The drawing under review shows one solid part. Ordinate dimensions are in mm from its lowest x, y, z. A direction names the side the tool comes from. Give positions to 0.01 mm unless a question says otherwise; leave off trailing zeros. Order: outer loops, then holes, each group sorted by start corner. A loop starts at its lowest first (then second) coordinate and runs counter-clockwise, first axis right, second up. Notation, with made-up numbers: (56, 19) -> (65, 19) arc R30 ccw to (65, 41) -> close; hole circle Ø7 at (-35, 32.5). An arc over 180 degrees is marked (long way). One line per item, written item: value. Start each with the question number.
1) Consider section D-D (x = 10). State the section outline as (y, z) points, plus the area to 3 significant figures.
2) Consider section A-A (x = 30). State the section outline as (y, z) points, plus the area to 3 significant figures.
3) Tool access review of the marked faces 4 and 5: name each direction out of +Z, -Z, +X, -X, +Y, -Y from which nothing blocks a thin tool from reaching the whole face with its end or side.
4) Consider section C-C (y = 16.5). State the section outline as (x, z) points, plus the area to 3 significant figures.
5) Wall thickness on line 1 along Z through (x, y) = (30, 14.5); line 2 along Y through (x, z) = (17, 3.5); line 3 along Z through (x, y) = (10, 15.75): over which ranges is each line inside the solid? List them lowest first. Write a range as from..to.
6) For pin 1 (4 mm diameter, centred on x = 30, z = 40.5, fed in from +Y); pin 2 (4 mm diameter, centred on x = 22, y = 69.5, fed in from -Z); pin 3 (1 mm diameter, centred on y = 68.5, z = 27.5, fed in from +X); pin 4 (6 mm diameter, centred on x = 30, z = 10, fed in from -Y), all flat-tipped, find the tip position at first contact; note any pin that passes through.
7) The part is to be moulded in two halves that separate along X. For the marked faces 1, 2 and 3, say which applies: released by +X, released by -X, zero draft, split by the parting line, or undercut.
8) Consider section B-B (z = 50). State the section outline as (x, y) points, plus the area to 3 significant figures.
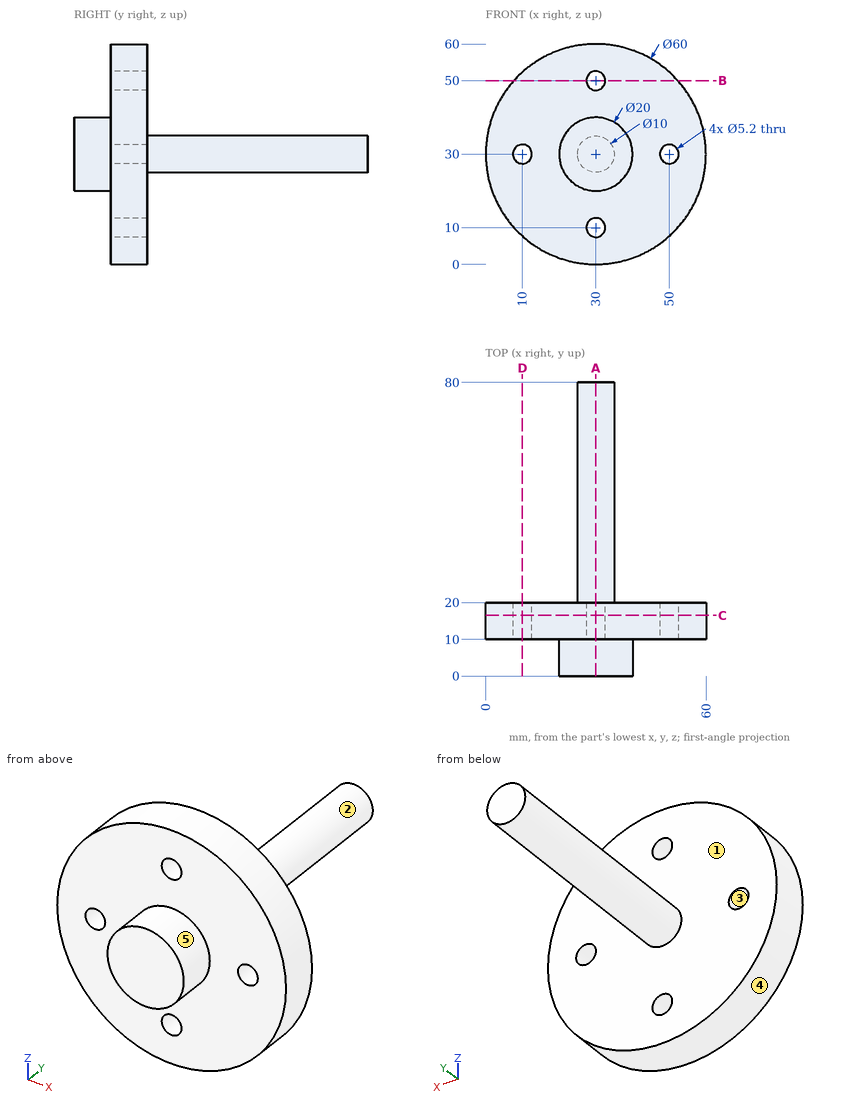
Checked values:
1. outline: (10, 7.64) -> (20, 7.64) -> (20, 27.4) -> (10, 27.4) -> close; (10, 32.6) -> (20, 32.6) -> (20, 52.36) -> (10, 52.36) -> close
1. area: 395 mm^2
2. outline: (0, 20) -> (10, 20) -> (10, 12.6) -> (20, 12.6) -> (20, 25) -> (80, 25) -> (80, 35) -> (20, 35) -> (20, 47.4) -> (10, 47.4) -> (10, 40) -> (0, 40) -> close; (10, 0) -> (20, 0) -> (20, 7.4) -> (10, 7.4) -> close; (10, 52.6) -> (20, 52.6) -> (20, 60) -> (10, 60) -> close
2. area: 1,300 mm^2
3. face 4: +Y, -Y
3. face 5: -Y
4. outline: circle Ø60 at (30, 30); hole circle Ø5.2 at (10, 30); hole circle Ø5.2 at (30, 10); hole circle Ø5.2 at (30, 50); hole circle Ø5.2 at (50, 30)
4. area: 2,740 mm^2
5. line 1: z = 0..7.4, 12.6..47.4, 52.6..60
5. line 2: y = 10..20
5. line 3: z = 7.64..27.4, 32.6..52.36
6. pin 1: stops at y = 20
6. pin 2: passes through
6. pin 3: stops at x = 34.58
6. pin 4: stops at y = 10
7. face 1: zero draft
7. face 2: split by the parting line
7. face 3: undercut
8. outline: (7.64, 10) -> (27.4, 10) -> (27.4, 20) -> (7.64, 20) -> close; (32.6, 10) -> (52.36, 10) -> (52.36, 20) -> (32.6, 20) -> close
8. area: 395 mm^2
